Could you check a few things on this model? Use its own coordinates, in mm. A direction names the side the tool comes from. Round coordinates to 2 decimals unless told otherwise and drop trailing zeros. Write each loop counter-clockwise with the first axis right and the second up, starting at its lowest first coordinate (ties: lowest second). Pieces come first, ordered by that corner, then holes.
```python
from build123d import *

# Parameters (mm, degrees)
PAD001_DEPTH = 20
SKETCH002_R  = 5.1
POCKET_DEPTH = 200
FILLET_R     = 6


with BuildPart() as part:
    # Sketch001 → Pad001 (new body)
    with BuildSketch(Plane.XY):
        Polygon((-70, 15), (-61.4, 15), (-61.4, 35), (-54, 35), (-54, 15), (54, 15), (54, 35), (61.4, 35), (61.4, 15), (70, 15), (70, 5.15), (61.079938, 10.3), (61.079938, -10.3), (70, -5.15), (70, -15), (-70, -15), (-70, -5), (-78.660254, -10), (-78.660254, 10), (-70, 5), align=None)
    extrude(amount=PAD001_DEPTH)

    # Sketch002 (on Face9 of Pad001) → Pocket (cut)
    with BuildSketch(Plane.YZ.offset(61.4)):
        with Locations((25, 10)):
            Circle(SKETCH002_R)
    extrude(amount=-POCKET_DEPTH, mode=Mode.SUBTRACT)

    # Fillet
    fillet_edges = [part.edges().sort_by_distance(p)[0] for p in [
        (57.7, 35, 20),
        (57.7, 35, 0),
        (-57.7, 35, 0),
        (-57.7, 35, 20),
    ]]
    fillet(fillet_edges, radius=FILLET_R)


solid = part.part
```
Q1. If I drill on L1, parallel to X at y = 17, z = 16.5; L2, parallel to Z at x = -56, y = 25; L3, parallel to X at y = -6.5, z = 4.75, over which ranges is the centre line in solid material (lowest first)?
Q2. I'm going to push flat-ended pins straight in: pin 1 Ø4.5 at (x, z) = (66, 5.5) entering from +Y; pin 2 Ø10 at (y, z) = (29, 9) entering from -X; pin 3 Ø6 at (y, z) = (25, 10) entering from -X; pin 4 Ø1.5 at (y, z) = (4.5, 10.5) entering from +X. Where does each tip first touch, or does it pass through?
Q3. We'd pull the mould along X, two halves only. Please class faces 5 (the flat face through (-58, 35, 10)), 6 (the flat face through (70, 10, 10)), 7 (the flat face through (-54, 27, 5)): pulls with the +X half, pulls with the -X half, needs draft (parallel to the pull), parting line crosses it, or undercut.
Q4. Imagine slicing it at C-C, the plane x = 3.5. Write out the boundary of the cut face in (y, z).
Q5. Imagine slicing it at B-B, the plane y = 25. Write out the boundary of the cut face in (x, z), then the cut area to 3 significant figures.
Q6. Imagine slicing it at A-A, the plane z = 10. Write out the boundary of the cut face in (x, y), then the cut area to 3 significant figures.
Q7. On a 3-axis mill with a long thin cutter (end or side, diameter ignored), from which of +Z, -Z, +X, -X, +Y, -Y can I reach the whole of each face in a straight line? I mean faces 1 (the flat face through (61.08, 0, 10)), 2 (the flat face through (-70, -10, 10)), 3 (the flat face through (66, 15, 10)), 4 (the flat face through (-70, 10, 10)). Say none if no direction works.
Results found:
1. L1: x = -61.4 to -54, 54 to 61.4
1. L2: z = 0 to 4.9, 15.1 to 20
1. L3: x = -78.66 to -72.6, -70 to 61.08, 67.66 to 70
2. pin 1: stops at y = 15
2. pin 2: stops at x = -61.4
2. pin 3: passes through
2. pin 4: stops at x = 70
3. face 5: needs draft
3. face 6: pulls with the +X half
3. face 7: undercut
4. outline: (-15, 0) - (15, 0) - (15, 20) - (-15, 20) - close
5. outline: (-61.4, 0) - (-54, 0) - (-54, 4.9) - (-61.4, 4.9) - close; (-61.4, 15.1) - (-54, 15.1) - (-54, 20) - (-61.4, 20) - close; (54, 0) - (61.4, 0) - (61.4, 4.9) - (54, 4.9) - close; (54, 15.1) - (61.4, 15.1) - (61.4, 20) - (54, 20) - close
5. area: 145 mm2
6. outline: (-78.66, -10) - (-70, -5) - (-70, -15) - (70, -15) - (70, -5.15) - (61.08, -10.3) - (61.08, 10.3) - (70, 5.15) - (70, 15) - (61.4, 15) - (61.4, 19.9) - (54, 19.9) - (54, 15) - (-54, 15) - (-54, 19.9) - (-61.4, 19.9) - (-61.4, 15) - (-70, 15) - (-70, 5) - (-78.66, 10) - close; (-61.4, 30.1) - (-54, 30.1) - (-54, 35) - (-61.4, 35) - close; (54, 30.1) - (61.4, 30.1) - (61.4, 35) - (54, 35) - close
6. area: 4,340 mm2
7. face 1: +Z, -Z
7. face 2: +Z, -Z, -Y
7. face 3: +Z, -Z, +X, +Y
7. face 4: +Z, -Z, +Y
